Geometry: see drawing. Coordinates: mm, zero at the bounding-box minimum. A direction names the side the tool comes from. Round coordinates to 2 decimals unless told otherwise and drop trailing zeros. Loops run counter-clockwise (first coordinate to the right, second up) from the corner with the lowest first, then second, coordinate; pieces in that order, holes last. Notation, with made-up numbers: M -30.5,89 L -18.5,89 A22 cw -18.5,110 Z; hole C 2,61.25 d4. An arc over 180 degrees is marked long. Answer as a JSON object with one key per item and string values.
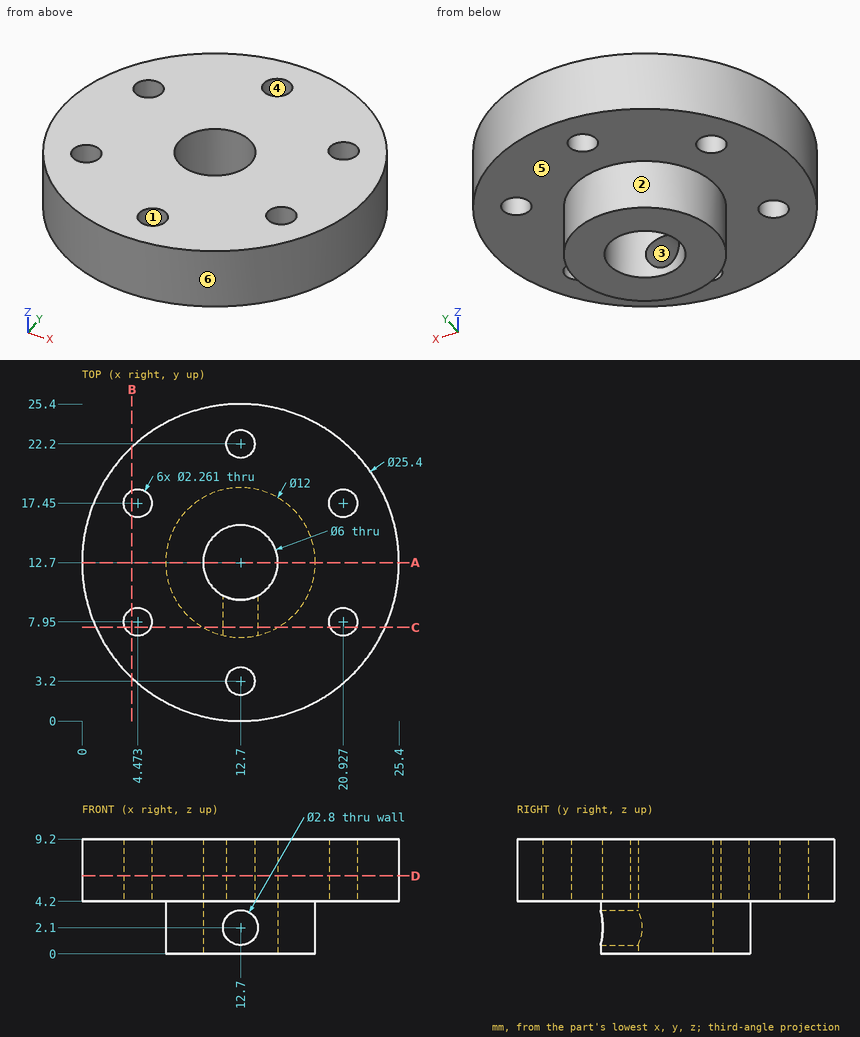
1) Pin query (flat end, axial travel): P1, Ø2, axis at x = 4.47, y = 17.45, coming from the -Z side; P2, Ø3, axis at y = 9.5, z = 5, coming from the -X side; P3, Ø1, axis at x = 9, z = 4, coming from the -Y side; P4, Ø3.5, axis at x = 20.93, y = 7.95, coming from the -Z side. Return the tip coordinate at first contact, or that it passes through.
Results:
{"P1": "through", "P2": "x = 0.11", "P3": "y = 0.42", "P4": "z = 4.2"}
2) Pull-direction query (Y, two-part tool) for the marked faces 4, 5 and 6; classes: +Y half, -Y half, draft (parallel to the pull), parting line (faces both ways), or undercut.
Results:
{"face 4": "undercut", "face 5": "draft", "face 6": "parting line"}
3) Section query D-D (z = 6.25). Return the cut outline in (x, y), and give its area (3 significant figures).
Results:
{"outline": "C 12.7,12.7 d25.4; hole C 4.47,7.95 d2.26; hole C 4.47,17.45 d2.26; hole C 12.7,12.7 d6; hole C 12.7,3.2 d2.26; hole C 12.7,22.2 d2.26; hole C 20.93,7.95 d2.26; hole C 20.93,17.45 d2.26", "area": "454 mm2"}
4) Section query A-A (y = 12.7). Return the cut outline in (x, z), and give its area (3 significant figures).
Results:
{"outline": "M 0,4.2 L 6.7,4.2 L 6.7,0 L 9.7,0 L 9.7,9.2 L 0,9.2 Z; M 15.7,0 L 18.7,0 L 18.7,4.2 L 25.4,4.2 L 25.4,9.2 L 15.7,9.2 Z", "area": "122 mm2"}
5) Reachability of the marked faces 1, 2 and 3 from +Z, -Z, +X, -X, +Y, -Y: full face, straight path, thin tool, end or side. Return the list, or none.
Results:
{"face 1": "+Z, -Z", "face 2": "-Z", "face 3": "-Y"}
6) Section query B-B (x = 4). Return the cut outline in (y, z).
Results:
{"outline": "M 3.45,4.2 L 6.92,4.2 L 6.92,9.2 L 3.45,9.2 Z; M 8.98,4.2 L 16.42,4.2 L 16.42,9.2 L 8.98,9.2 Z; M 18.48,4.2 L 21.95,4.2 L 21.95,9.2 L 18.48,9.2 Z"}
7) Ray query, line 1 (Y direction, x = 12.7, z = 7.4); line 2 (X direction, y = 8.25, z = 6) (1 decimal); line 3 (Y direction, x = 5.5, z = 5.75) (1 decimal). Return the intervals inside material, ascending.
Results:
{"line 1": "0 to 2.07, 4.33 to 9.7, 15.7 to 21.07, 23.33 to 25.4", "line 2": "0.8 to 3.4, 5.6 to 19.8, 22 to 24.6", "line 3": "2.2 to 7.5, 8.4 to 17, 17.9 to 23.2"}
8) Section query C-C (y = 7.5). Return the cut outline in (x, z), and give its area (3 significant figures).
Results:
{"outline": "M 1.11,4.2 L 3.44,4.2 L 3.44,9.2 L 1.11,9.2 Z; M 5.51,4.2 L 9.71,4.2 L 9.71,0 L 15.69,0 L 15.69,4.2 L 19.89,4.2 L 19.89,9.2 L 5.51,9.2 Z; M 21.96,4.2 L 24.29,4.2 L 24.29,9.2 L 21.96,9.2 Z; hole C 12.7,2.1 d2.8", "area": "114 mm2"}
